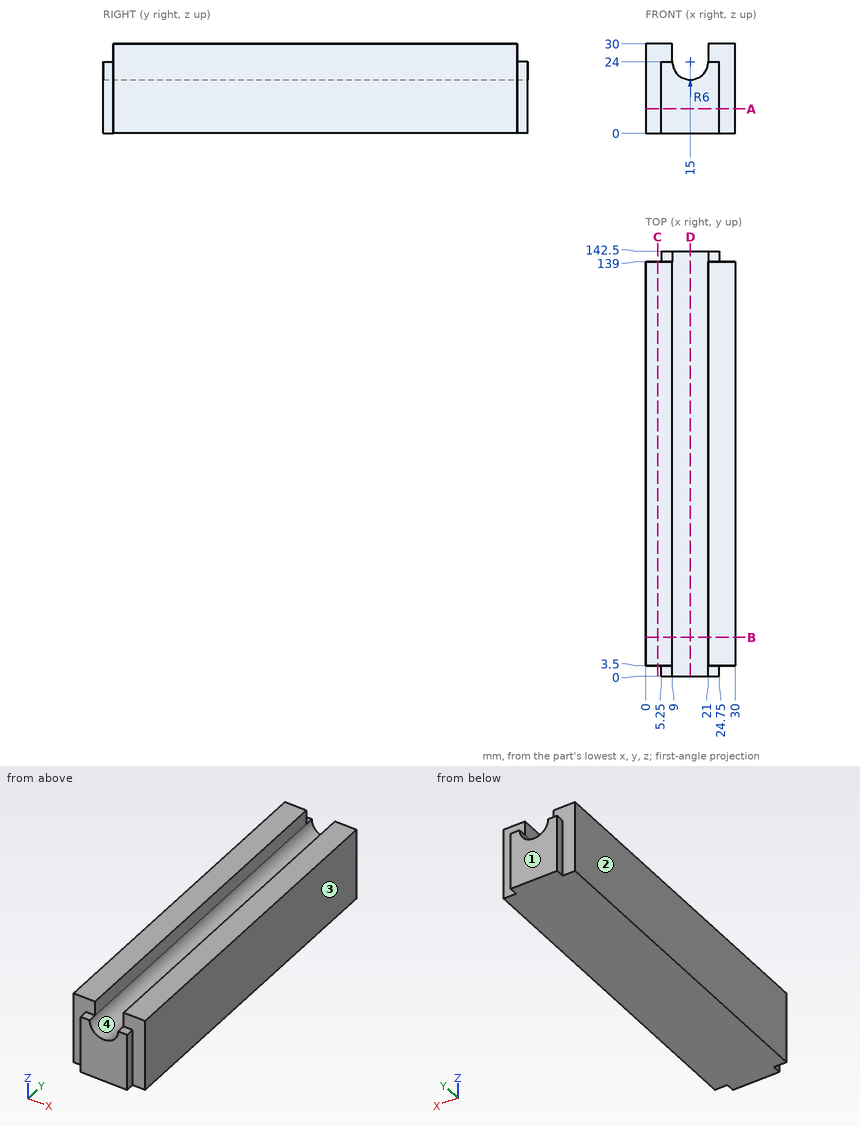
Answer from the drawing. Dimensions are ordinates in mm from the lowest x, y and z of the part. Coordinates: 2 decimals unless noted, no trailing zeros. Loops run counter-clockwise (first coordinate to the right, second up) from the corner with the lowest first, then second, coordinate; pieces in that order, holes last.
Q1. The mould has two halves that part along X. Classify the marked faces 1, 2, 3 and 4: +X half, -X half, draft (parallel to the pull), parting line (faces both ways), or undercut.
Q2. The part is cut by section B-B on y = 13. Write down the section's boundary in (x, z).
Q3. The part is cut by section C-C on x = 4. Write down the section's boundary in (y, z), and give its area (4 significant figures).
Q4. Each of these flat-tipped pins is pushed along its axis until it touches: pin 1 Ø4 at (y, z) = (2.5, 14.5) entering from +X; pin 2 Ø1 at (y, z) = (1.5, 14) entering from -X; pin 3 Ø1.5 at (x, y) = (14.5, 119.5) entering from +Z; pin 4 Ø3 at (x, y) = (22, 141) entering from +Z. Where does it stop, or does it pass through?
Q5. Consider probe 1 along X at (y, z) = (126, 26.25); probe 2 along Y at (x, z) = (26.5, 11); probe 3 along Z at (x, y) = (15.25, 36.5). Determine where each line is inside the solid, lowest interval first.
Q6. The part is cut by section D-D on x = 15. Write down the section's boundary in (y, z).
Q7. The part is cut by section A-A on z = 8.25. Write down the section's boundary in (x, y).
Results below:
1. face 1: draft
1. face 2: -X half
1. face 3: +X half
1. face 4: undercut
2. outline: (0, 0) - (30, 0) - (30, 30) - (21, 30) - (21, 24) arc R6 cw to (9, 24) - (9, 30) - (0, 30) - close
3. outline: (3.5, 0) - (139, 0) - (139, 30) - (3.5, 30) - close
3. area: 4,065 mm2
4. pin 1: stops at x = 30
4. pin 2: stops at x = 5.25
4. pin 3: stops at z = 18.13
4. pin 4: stops at z = 24
5. probe 1: x = 0 to 9, 21 to 30
5. probe 2: y = 3.5 to 139
5. probe 3: z = 0 to 18.01
6. outline: (0, 0) - (142.5, 0) - (142.5, 18) - (0, 18) - close
7. outline: (0, 3.5) - (5.25, 3.5) - (5.25, 0) - (24.75, 0) - (24.75, 3.5) - (30, 3.5) - (30, 139) - (24.75, 139) - (24.75, 142.5) - (5.25, 142.5) - (5.25, 139) - (0, 139) - close
